Geometry check sheet. Reference: the model listing, model coordinates, mm. Round coordinates to 2 decimals unless told otherwise and drop trailing zeros. Order: outer loops, then holes, each group sorted by start corner. A loop starts at its lowest first (then second) coordinate and runs counter-clockwise, first axis right, second up. Notation, with made-up numbers: (9.5, -9.5) - (65.5, -9.5) arc R15 ccw to (65.5, 15.5) - close; hole circle Ø11 at (-31, 56.25). An arc over 180 degrees is marked (long way). One line per question, with ' | ' between items. Start each with the question number.
Q1. Sectioned sample at B-B, the plane y = -18.5. Enter the section's corners in (x, z), then the cut area to 3 significant figures.
Q2. Sectioned sample at A-A, the plane x = -13. Enter the section's corners in (y, z).
Q3. Gauge pin test, flat end, axial feed: P1, Ø3, axis at x = -13, y = -18.5, coming from the -Z side. Record the tip position at first contact, or that the pin passes through.
Q4. Sectioned sample at D-D, the plane y = 17.5. Enter the section's corners in (x, z).
Q5. Material ranges on line 1 along Y through (x, z) = (-13, 0.3); line 2 along Y through (x, z) = (10, 2); line 3 along X through (y, z) = (-19, 2.2), recorded low to high.
Q6. Sectioned sample at C-C, the plane z = 1.2. Enter the section's corners in (x, y), then the cut area to 3 significant figures.
```python
from build123d import *

# Parameters (mm, degrees)
F0_R     = 1.25
F1_DEPTH = 2.5
F2_R     = 2


with BuildPart() as f1:
    # F0 (on Top) → F1 (new body)
    with BuildSketch(Plane.XY):
        Polygon((8.5, 15), (8.5, -16), (5, -16), (5, -21), (13.5, -21), (13.5, 20), (-15.5, 20), (-15.5, -21), (-7, -21), (-7, -16), (-10.5, -16), (-10.5, 15), align=None)
        with Locations((-13, -18.5)):
            Circle(F0_R, mode=Mode.SUBTRACT)
        with Locations((11, -18.5)):
            Circle(F0_R, mode=Mode.SUBTRACT)
        with Locations((-13, 17.5)):
            Circle(F0_R, mode=Mode.SUBTRACT)
        with Locations((11, 17.5)):
            Circle(F0_R, mode=Mode.SUBTRACT)
        Polygon((5, -16), (8.5, -16), (8.5, 15), (-10.5, 15), (-10.5, -16), (-7, -16), align=None)
    extrude(amount=F1_DEPTH)

    # F2
    f2_edges = [f1.edges().sort_by_distance(p)[0] for p in [
        (-15.5, 20, 1.25),
        (13.5, 20, 1.25),
        (13.5, -21, 1.25),
        (-15.5, -21, 1.25),
    ]]
    fillet(f2_edges, radius=F2_R)


solid = f1.part
```
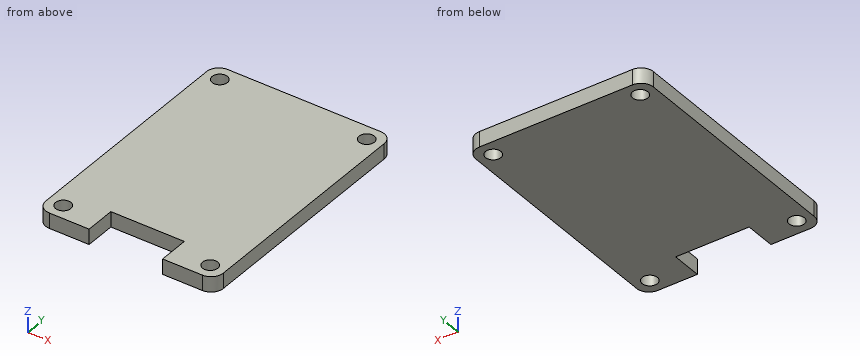
Determined:
1) outline: (-15.5, 0) - (-14.25, 0) - (-14.25, 2.5) - (-15.5, 2.5) - close; (-11.75, 0) - (-7, 0) - (-7, 2.5) - (-11.75, 2.5) - close; (5, 0) - (9.75, 0) - (9.75, 2.5) - (5, 2.5) - close; (12.25, 0) - (13.5, 0) - (13.5, 2.5) - (12.25, 2.5) - close | area: 30.0 mm2
2) outline: (-21, 0) - (-19.75, 0) - (-19.75, 2.5) - (-21, 2.5) - close; (-17.25, 0) - (16.25, 0) - (16.25, 2.5) - (-17.25, 2.5) - close; (18.75, 0) - (20, 0) - (20, 2.5) - (18.75, 2.5) - close
3) P1: stops at z = 0
4) outline: (-15.5, 0) - (-14.25, 0) - (-14.25, 2.5) - (-15.5, 2.5) - close; (-11.75, 0) - (9.75, 0) - (9.75, 2.5) - (-11.75, 2.5) - close; (12.25, 0) - (13.5, 0) - (13.5, 2.5) - (12.25, 2.5) - close
5) line 1: y = -21 to -19.75, -17.25 to 16.25, 18.75 to 20 | line 2: y = -21 to -19.25, -17.75 to 16.75, 18.25 to 20 | line 3: x = -15.5 to -14.15, -11.85 to -7, 5 to 9.85, 12.15 to 13.5
6) outline: (-15.5, -19) arc R2 ccw to (-13.5, -21) - (-7, -21) - (-7, -16) - (5, -16) - (5, -21) - (11.5, -21) arc R2 ccw to (13.5, -19) - (13.5, 18) arc R2 ccw to (11.5, 20) - (-13.5, 20) arc R2 ccw to (-15.5, 18) - close; hole circle Ø2.5 at (-13, -18.5); hole circle Ø2.5 at (-13, 17.5); hole circle Ø2.5 at (11, -18.5); hole circle Ø2.5 at (11, 17.5) | area: 1,110 mm2
